Geometry check sheet. Reference: the model listing, model coordinates, mm. Give positions to 0.01 mm unless a question says otherwise; leave off trailing zeros. Order: outer loops, then holes, each group sorted by start corner. A loop starts at its lowest first (then second) coordinate and runs counter-clockwise, first axis right, second up. Notation, with made-up numbers: M 34,-37.75 L 88,-37.75 A20 cw 88,-15.75 Z; hole C 43,-23 d3. An arc over 180 degrees is marked long. Use CSV: the item, a comma, the result in double quotes. Start each with the question number.
Autodesk Inventor part; units mm, degrees
ref_plane "YZ Plane" through (0, 0, 0) normal (1, 0, 0) x (0, 1, 0)
ref_plane "XZ Plane" through (0, 0, 0) normal (0, 1, 0) x (-1, 0, 0)
ref_plane "XY Plane" through (0, 0, 0) normal (0, 0, 1) x (1, 0, 0)
sketch "Sketch1" plane through (0, 0, 0) normal (0, 0, 1) x (1, 0, 0)
  line L0 (13.75, 44.8) -> (-36.25, 44.8)
  line L1 (-36.25, 44.8) -> (-36.25, -55.2)
  line L2 (-36.25, -55.2) -> (13.75, -55.2)
  line L3 (13.75, -55.2) -> (13.75, 44.8)
  circle A0 centre (-2.5, -5.2) radius 2.5 construction
  circle A1 centre (-20, -5.2) radius 2.5 construction
  circle A2 centre (-11.25, -39.5) radius 2.5 construction
  circle A3 centre (-2.5, -5.2) radius 3.25
  circle A4 centre (-20, -5.2) radius 3.25
  circle A5 centre (-11.25, -39.5) radius 3.25
  point P0 (0, 0)
  dimension "d0" = 6.5
  dimension "d1" = 6.5
  dimension "d2" = 6.5
extrude "Extrusion1" add sketch "Sketch1" along normal blind 3.4
properties part number "Motor cover upper"
(1) Sectioned sample at C-C on y = -39.5. Record the cut outline in (x, z), then the cut area to 3 significant figures.
(2) Draft check along X on faces 1 (the face through (-12, -55.2, 2)), 2 (the face through (-23.247, -5.343, 1.676)), 3 (the face through (-36.25, -5, 2)), 4 (the face through (13.75, -6, 2)). Enter one of: +X half, -X half, draft (parallel to the pull), parting line (faces both ways), or undercut.
(3) Sectioned sample at D-D on y = -5.2. Record the cut outline in (x, z).
(4) Sectioned sample at B-B on z = 2.8. Record the cut outline in (x, y), then the cut area to 3 significant figures.
(5) Thickness scan on line 1 (Y direction, x = -11, z = 2.2); line 2 (Y direction, x = -20, z = 1.6). Record the ranges inside material, lowest first.
(6) Sectioned sample at A-A on x = -2.5. Record the cut outline in (y, z), then the cut area to 3 significant figures.
Responses:
1,outline,"M -36.25,0 L -14.5,0 L -14.5,3.4 L -36.25,3.4 Z; M -8,0 L 13.75,0 L 13.75,3.4 L -8,3.4 Z"
1,area,"148 mm2"
2,face 1,"draft"
2,face 2,"undercut"
2,face 3,"-X half"
2,face 4,"+X half"
3,outline,"M -36.25,0 L -23.25,0 L -23.25,3.4 L -36.25,3.4 Z; M -16.75,0 L -5.75,0 L -5.75,3.4 L -16.75,3.4 Z; M 0.75,0 L 13.75,0 L 13.75,3.4 L 0.75,3.4 Z"
4,outline,"M -36.25,-55.2 L 13.75,-55.2 L 13.75,44.8 L -36.25,44.8 Z; hole C -20,-5.2 d6.5; hole C -11.25,-39.5 d6.5; hole C -2.5,-5.2 d6.5"
4,area,"4,900 mm2"
5,line 1,"-55.2 to -42.74, -36.26 to 44.8"
5,line 2,"-55.2 to -8.45, -1.95 to 44.8"
6,outline,"M -55.2,0 L -8.45,0 L -8.45,3.4 L -55.2,3.4 Z; M -1.95,0 L 44.8,0 L 44.8,3.4 L -1.95,3.4 Z"
6,area,"318 mm2"
